Input: part model. Units: mm. Frame: model coordinates. Face numbers are marked on the shaded views. A direction names the side the tool comes from. Round coordinates to 2 decimals unless told otherwise and drop trailing zeros. Order: outer loops, then holes, each group sorted by start corner. A loop starts at its lowest first (then second) coordinate and runs counter-clockwise, first axis right, second up. Notation, with made-up numbers: (-3, 52) -> (34, 52) arc R17 ccw to (34, 73) -> close; hole circle Ø9 at (74.25, 35.5). An arc over 180 degrees is marked (long way). Use a Markdown table: item, result.
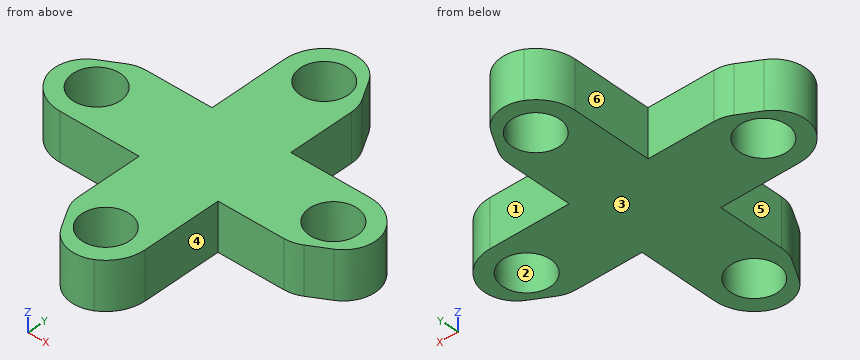
Autodesk Inventor part; units mm, degrees
ref_plane "YZ Plane" through (0, 0, 0) normal (1, 0, 0) x (0, 1, 0)
ref_plane "XZ Plane" through (0, 0, 0) normal (0, 1, 0) x (-1, 0, 0)
ref_plane "XY Plane" through (0, 0, 0) normal (0, 0, 1) x (1, 0, 0)
sketch "스케치1" plane through (0, 0, 0) normal (0, 0, 1) x (1, 0, 0)
  circle A0 centre (0, 0) radius 9.9
  arc A1 (-2.475, 0) -> (2.475, 0) centre (0, 0) ccw
  arc A2 (2.475, 7.425) -> (-2.475, 7.425) centre (0, 7.425) ccw
  line L0 (-2.475, 7.425) -> (-2.475, 0)
  line L1 (2.475, 7.425) -> (2.475, 0)
  arc A3 (-7.425, 2.475) -> (-7.425, -2.475) centre (-7.425, 0) ccw
  line L2 (-7.425, 2.475) -> (0, 2.475)
  line L3 (-7.425, -2.475) -> (0, -2.475)
  arc A4 (0, -2.475) -> (0, 2.475) centre (0, 0) ccw
  arc A5 (-2.475, -7.425) -> (2.475, -7.425) centre (0, -7.425) ccw
  line L4 (-2.475, -7.425) -> (-2.475, 0)
  line L5 (2.475, -7.425) -> (2.475, 0)
  arc A6 (2.475, 0) -> (-2.475, 0) centre (0, 0) ccw
  arc A7 (7.425, -2.475) -> (7.425, 2.475) centre (7.425, 0) ccw
  line L6 (7.425, -2.475) -> (0, -2.475)
  line L7 (7.425, 2.475) -> (0, 2.475)
  arc A8 (0, 2.475) -> (0, -2.475) centre (0, 0) ccw
  point P0 (-2.475, 2.475)
  point P1 (-2.475, -2.475)
  point P2 (2.475, -2.475)
  point P3 (2.475, 2.475)
  dimension "d0" = 19.8
  dimension "d1" = 4.95
  dimension "d2" = 4.95
  dimension "d5" = 360
extrude "돌출1" add sketch "스케치1" along normal blind 3 contours A7 L6 L5 L1 L7 | A2 L1 L7 L2 L0 | A5 L4 L3 L6 L5 | A3 L2 L0 L4 L3 | L6 A1 L5 | L1 A4 L7 | L2 A6 L0 | L4 A1 L3 | A1 A6 A4
sketch "스케치2" plane through (0, 0, 3) normal (0, 0, 1) x (1, 0, 0)
  arc A0 (2.475, 7.425) -> (-2.475, 7.425) centre (0, 7.425) ccw
  circle A1 centre (0, 7.425) radius 1.5
  point P0 (0, 0)
  dimension "d9" = 3
extrude "돌출2" cut sketch "스케치2" against normal through all
pattern_circular "원형 패턴1" count 4 over 360 about axis through (0, 0, -10) along (0, 0, 1) of "돌출2"
sketch "스케치3" plane through (0, 0, 3) normal (0, 0, 1) x (1, 0, 0)
  arc A0 (2.475, 7.425) -> (-2.475, 7.425) centre (0, 7.425) ccw
  line L0 (1, 9.689) -> (2.475, 7.1422)
  line L1 (2.475, 2.475) -> (2.475, 7.425)
  circle A1 centre (0, 7.425) radius 1.5
  point P0 (0, 0)
  dimension "d15" = 0.5
  dimension "d16" = 1
extrude "돌출3" cut sketch "스케치3" against normal through all contours L1 L0 A0
fillet "모깎기1" radius 2 1 edges at (1, 9.689, 1.5)
fillet "모깎기2" radius 2 1 edges at (2.475, 7.1422, 1.5)
pattern_circular "원형 패턴2" count 4 over 360 about axis through (0, 0, -10) along (0, 0, 1) of "돌출3", "모깎기1", "모깎기2"
equation "\"d1\" = 0.25 * d0"
equation "\"d2\" = d1"
properties part number "ModuleConnector_Center_Axis_3D 인쇄"
1) Cut plane A-A on z = 2.4. Return loops of the section in (x, y) (3 decimals), and give its area (3 significant figures).
Results found:
| item | result |
|---|---|
| outline | (-9.567, -1.24) arc R2.475 ccw to (-7.425, -2.475) -> (-2.475, -2.475) -> (-2.475, -6.605) arc R2 ccw to (-2.206, -7.607) -> (-1.493, -8.838) arc R2 ccw to (1.24, -9.567) arc R2.475 ccw to (2.475, -7.425) -> (2.475, -2.475) -> (6.605, -2.475) arc R2 ccw to (7.607, -2.206) -> (8.838, -1.493) arc R2 ccw to (9.567, 1.24) arc R2.475 ccw to (7.425, 2.475) -> (2.475, 2.475) -> (2.475, 6.605) arc R2 ccw to (2.206, 7.607) -> (1.493, 8.838) arc R2 ccw to (-1.24, 9.567) arc R2.475 ccw to (-2.475, 7.425) -> (-2.475, 2.475) -> (-6.605, 2.475) arc R2 ccw to (-7.607, 2.206) -> (-8.838, 1.493) arc R2 ccw to start; hole circle Ø3 at (-7.425, 0); hole circle Ø3 at (0, -7.425); hole circle Ø3 at (0, 7.425); hole circle Ø3 at (7.425, 0) |
| area | 128 mm² |
2) Pin query (flat end, axial travel): pin 1 Ø0.9 at (x, z) = (5.5, 1.5) entering from +Y (3 decimals); pin 2 Ø4 at (x, y) = (0, 7.425) entering from +Z; pin 3 Ø0.9 at (x, z) = (-6, 1.5) entering from -Y (3 decimals); pin 4 Ø1.5 at (y, z) = (-3.5, 1.5) entering from -X (3 decimals). Return the tip coordinate at first contact, or that it passes through.
Results found:
| item | result |
|---|---|
| pin 1 | stops at y = 2.475 |
| pin 2 | stops at z = 3 |
| pin 3 | stops at y = -2.475 |
| pin 4 | stops at x = -2.475 |
3) Cut plane B-B on y = 0. Return loops of the section in (x, z) (3 decimals).
Results found:
| item | result |
|---|---|
| outline | (-9.822, 0) -> (-8.925, 0) -> (-8.925, 3) -> (-9.822, 3) -> close; (-5.925, 0) -> (5.925, 0) -> (5.925, 3) -> (-5.925, 3) -> close; (8.925, 0) -> (9.822, 0) -> (9.822, 3) -> (8.925, 3) -> close |
4) Set-up query: the marked faces 4, 5 and 6. Return all of +Z, -Z, +X, -X, +Y, -Y with unobstructed straight access to the full face (end or side cutting, diameter ignored); none if empty.
Results found:
| item | result |
|---|---|
| face 4 | +Z, -Z, +X, -Y |
| face 5 | +Z, -Z, -X, -Y |
| face 6 | +Z, -Z, -X, +Y |
5) Cut plane D-D on y = -8.5. Return loops of the section in (x, z).
Results found:
| item | result |
|---|---|
| outline | (-1.69, 0) -> (-1.05, 0) -> (-1.05, 3) -> (-1.69, 3) -> close; (1.05, 0) -> (2.23, 0) -> (2.23, 3) -> (1.05, 3) -> close |
6) Pull-direction query (Y, two-part tool) for the marked faces 1, 2 and 3; classes: +Y half, -Y half, draft (parallel to the pull), parting line (faces both ways), or undercut.
Results found:
| item | result |
|---|---|
| face 1 | +Y half |
| face 2 | undercut |
| face 3 | draft |
7) Line query: L1, parallel to X at y = 0, z = 0.7 (3 decimals); L2, parallel to X at y = 4.75, z = 2.7 (3 decimals). Output: solid intervals per line, ascending. Write a range as [from, to].
Results found:
| item | result |
|---|---|
| L1 | x = [-9.822, -8.925], [-5.925, 5.925], [8.925, 9.822] |
| L2 | x = [-2.475, 2.475] |
